Geometry check sheet. Reference: the model listing, model coordinates, mm. A direction names the side the tool comes from. Coordinates: 2 decimals unless noted, no trailing zeros. Order: outer loops, then holes, each group sorted by start corner. A loop starts at its lowest first (then second) coordinate and runs counter-clockwise, first axis right, second up. Notation, with made-up numbers: (67.5, -10.5) -> (125.5, -10.5) arc R11 cw to (125.5, -3.5) -> close; hole circle Ø10 at (-17.5, 77.25). An arc over 180 degrees is marked (long way). Answer in a Markdown table with one row per item. Add a question column.
```python
from build123d import *

# Parameters (mm, degrees)
SKETCH1_W           = 157.48
SKETCH1_H           = 106.68
BOSS_EXTRUDE1_DEPTH = 49.784
SKETCH3_W           = 152.4
SKETCH3_H           = 101.6
CUT_EXTRUDE1_DEPTH  = 44.704
SKETCH4_W           = 8.89
SKETCH4_H           = 12.7
CUT_EXTRUDE2_DEPTH  = 43.18
SKETCH6_W           = 9.525
SKETCH6_H           = 12.7
CUT_EXTRUDE3_DEPTH  = 43.18


with BuildPart() as part:
    # Sketch1 → Boss-Extrude1 (new body)
    with BuildSketch(Plane.XY):
        Rectangle(SKETCH1_W, SKETCH1_H)
    extrude(amount=BOSS_EXTRUDE1_DEPTH)

    # Sketch3 → Cut-Extrude1 (cut)
    with BuildSketch(Plane.XY.offset(49.784)):
        Rectangle(SKETCH3_W, SKETCH3_H)
    extrude(amount=-CUT_EXTRUDE1_DEPTH, mode=Mode.SUBTRACT)

    # Sketch4 → Cut-Extrude2 (cut)
    with BuildSketch(Plane(origin=(78.74, 0, 0), x_dir=(0, 0, -1), z_dir=(1, 0, 0))):
        with Locations((-32.385, -8.89)):
            Rectangle(SKETCH4_W, SKETCH4_H)
    extrude(amount=-CUT_EXTRUDE2_DEPTH, mode=Mode.SUBTRACT)

    # Sketch6 → Cut-Extrude3 (cut)
    with BuildSketch(Plane.ZY.offset(78.74)):
        with Locations((35.2425, -21.59)):
            Rectangle(SKETCH6_W, SKETCH6_H)
    extrude(amount=-CUT_EXTRUDE3_DEPTH, mode=Mode.SUBTRACT)


solid = part.part
```
(1) Go/stop test with a flat-tipped pin: P1, Ø1, axis at x = 28.5, y = 36, coming from the +Z side. Record where the tip stops, or that it passes through.
(2) Cross-section at B-B (y = -23). Enter the section's corners in (x, z) (3 decimals).
(3) Access from +Z, -Z, +X, -X, +Y, -Y to the whole of each face (thin tool, end or side, straight path). Record for faces 5 (the face through (-76.2, -1, 28)), 6 (the face through (0, 52, 49.784)).
(4) Cross-section at A-A (z = 19). Enter the section's corners in (x, y).
(5) Scan lines: line 1 along X through (y, z) = (-30, 45); line 2 along Y through (x, z) = (-43, 16); line 3 along Z through (x, y) = (-40, 7). Record each from-to range of solid material in increasing order.
(6) Mould release check, pull along Y, two halves, no side actions. Record for faces 1 (the face through (-1, -53.34, 25)), 2 (the face through (-1, 1, 0)), 3 (the face through (-1, 53.34, 25)), 4 (the face through (-1, 1, 5.08)): +Y half, -Y half, draft (parallel to the pull), parting line (faces both ways), or undercut.
(7) Cross-section at D-D (x = 47). Enter the section's corners in (y, z).
(8) Cross-section at C-C (z = 33). Enter the section's corners in (x, y), plus the area to 3 significant figures.
Checks:
| question | item | result |
|---|---|---|
| 1 | P1 | z = 5.08 |
| 2 | outline | (-78.74, 0) -> (78.74, 0) -> (78.74, 49.784) -> (76.2, 49.784) -> (76.2, 5.08) -> (-76.2, 5.08) -> (-76.2, 30.48) -> (-78.74, 30.48) -> close; (-78.74, 40.005) -> (-76.2, 40.005) -> (-76.2, 49.784) -> (-78.74, 49.784) -> close |
| 3 | face 5 | +Z |
| 3 | face 6 | +Z, +X, -X, +Y, -Y |
| 4 | outline | (-78.74, -53.34) -> (78.74, -53.34) -> (78.74, 53.34) -> (-78.74, 53.34) -> close; hole (-76.2, -50.8) -> (76.2, -50.8) -> (76.2, 50.8) -> (-76.2, 50.8) -> close |
| 5 | line 1 | -78.74 to -76.2, 76.2 to 78.74 |
| 5 | line 2 | -53.34 to -50.8, 50.8 to 53.34 |
| 5 | line 3 | 0 to 5.08 |
| 6 | face 1 | -Y half |
| 6 | face 2 | draft |
| 6 | face 3 | +Y half |
| 6 | face 4 | undercut |
| 7 | outline | (-53.34, 0) -> (53.34, 0) -> (53.34, 49.78) -> (50.8, 49.78) -> (50.8, 5.08) -> (-50.8, 5.08) -> (-50.8, 49.78) -> (-53.34, 49.78) -> close |
| 8 | outline | (-78.74, -53.34) -> (78.74, -53.34) -> (78.74, -15.24) -> (76.2, -15.24) -> (76.2, -50.8) -> (-76.2, -50.8) -> (-76.2, -27.94) -> (-78.74, -27.94) -> close; (-78.74, -15.24) -> (-76.2, -15.24) -> (-76.2, 50.8) -> (76.2, 50.8) -> (76.2, -2.54) -> (78.74, -2.54) -> (78.74, 53.34) -> (-78.74, 53.34) -> close |
| 8 | area | 1,250 mm² |
